```python
from build123d import *

# Parameters (mm, degrees)
SKIZZE1_W                        = 266
SKIZZE1_H                        = 80
AUFSATZ_LINEAR_AUSTRAGEN1_DEPTH  = 20
SKIZZE4_R                        = 6.5
SCHNITT_LINEAR_AUSTRAGEN1_DEPTH  = 20
SKIZZE9_R                        = 15
SCHNITT_LINEAR_AUSTRAGEN5_DEPTH  = 16.8
SKIZZE10_W                       = 20
SKIZZE10_H                       = 15
SCHNITT_LINEAR_AUSTRAGEN6_DEPTH  = 24.3
SKIZZE11_W                       = 91.383535354
SKIZZE11_H                       = 106.650454953
SKIZZE11_W_2                     = 30.220228655
SKIZZE11_H_2                     = 75
SCHNITT_LINEAR_AUSTRAGEN7_DEPTH  = 304.3
SKIZZE12_R                       = 24.75
SCHNITT_LINEAR_AUSTRAGEN8_DEPTH  = 3
SKIZZE13_W                       = 20
SKIZZE13_H                       = 20
SCHNITT_LINEAR_AUSTRAGEN10_DEPTH = 20
VERRUNDUNG1_R                    = 3
SKIZZE14_W                       = 20
SKIZZE14_H                       = 20
SCHNITT_LINEAR_AUSTRAGEN11_DEPTH = 20
VERRUNDUNG2_R                    = 3
SKIZZE15_R                       = 2
SCHNITT_LINEAR_AUSTRAGEN12_DEPTH = 20
M5_GEWINDEBOHRUNG1_D             = 4.2
M5_GEWINDEBOHRUNG1_CSINK_D       = 5.05
M5_GEWINDEBOHRUNG1_CSINK_ANGLE   = 90
SCHNITT_LINEAR_AUSTRAGEN13_DEPTH = 30
SCHNITT_LINEAR_AUSTRAGEN14_DEPTH = 6
SKIZZE19_R                       = 3
SCHNITT_LINEAR_AUSTRAGEN15_DEPTH = 20


with BuildPart() as part:
    # Skizze1 → Aufsatz-Linear austragen1 (new body)
    with BuildSketch(Plane.XY):
        with Locations((43.523698588, -6.755674232)):
            Rectangle(SKIZZE1_W, SKIZZE1_H)
    extrude(amount=AUFSATZ_LINEAR_AUSTRAGEN1_DEPTH)

    # Skizze4 → Schnitt-Linear austragen1 (cut)
    with BuildSketch(Plane(origin=(0, 0, 0), x_dir=(-1, 0, 0), z_dir=(0, 0, -1))):
        with Locations((-43.523698588, -6.755674232)):
            Circle(SKIZZE4_R)
    extrude(amount=-SCHNITT_LINEAR_AUSTRAGEN1_DEPTH, mode=Mode.SUBTRACT)

    # Skizze9 → Schnitt-Linear austragen5 (cut)
    with BuildSketch(Plane(origin=(0, 0, 0), x_dir=(-1, 0, 0), z_dir=(0, 0, -1))):
        with Locations((-43.523698588, -6.755674232)):
            Circle(SKIZZE9_R)
    extrude(amount=-SCHNITT_LINEAR_AUSTRAGEN5_DEPTH, mode=Mode.SUBTRACT)

    # Skizze10 → Schnitt-Linear austragen6 (cut)
    with BuildSketch(Plane.XY.offset(20)):
        with Locations((-79.476301412, 25.744325768)):
            Rectangle(SKIZZE10_W, SKIZZE10_H)
        with Locations((-79.476301412, -39.255674232)):
            Rectangle(SKIZZE10_W, SKIZZE10_H)
        with Locations((166.523698588, -39.255674232)):
            Rectangle(SKIZZE10_W, SKIZZE10_H)
        with Locations((166.523698588, 25.744325768)):
            Rectangle(SKIZZE10_W, SKIZZE10_H)
    extrude(amount=-SCHNITT_LINEAR_AUSTRAGEN6_DEPTH, mode=Mode.SUBTRACT)

    # Skizze11 → Schnitt-Linear austragen7 (cut)
    with BuildSketch(Plane.ZY.offset(89.476301412)):
        with Locations((10.152146704, -6.755674232)):
            Rectangle(SKIZZE11_W, SKIZZE11_H)
        with Locations((10.152146705, -6.755674232)):
            Rectangle(SKIZZE11_W_2, SKIZZE11_H_2, mode=Mode.SUBTRACT)
    extrude(amount=-SCHNITT_LINEAR_AUSTRAGEN7_DEPTH, mode=Mode.SUBTRACT)

    # Skizze12 → Schnitt-Linear austragen8 (cut)
    with BuildSketch(Plane(origin=(0, 0, 0), x_dir=(-1, 0, 0), z_dir=(0, 0, -1))):
        with Locations((-43.523698588, -6.755674232)):
            Circle(SKIZZE12_R)
    extrude(amount=-SCHNITT_LINEAR_AUSTRAGEN8_DEPTH, mode=Mode.SUBTRACT)

    # Skizze13 → Schnitt-Linear austragen10 (cut)
    with BuildSketch(Plane.ZY.offset(89.476301412)):
        with Locations((10, -6.755674232)):
            Rectangle(SKIZZE13_W, SKIZZE13_H)
    extrude(amount=-SCHNITT_LINEAR_AUSTRAGEN10_DEPTH, mode=Mode.SUBTRACT)

    # Verrundung1
    verrundung1_edges = [part.edges().sort_by_distance(p)[0] for p in [
        (-69.476301412, 3.244325768, 10),
        (-69.476301412, -16.755674232, 10),
        (-69.476301412, -31.755674232, 10),
        (-69.476301412, 18.244325768, 10),
    ]]
    fillet(verrundung1_edges, radius=VERRUNDUNG1_R)

    # Skizze14 → Schnitt-Linear austragen11 (cut)
    with BuildSketch(Plane(origin=(176.523698588, 0, 0), x_dir=(0, 0, -1), z_dir=(1, 0, 0))):
        with Locations((-10, -6.755674232)):
            Rectangle(SKIZZE14_W, SKIZZE14_H)
    extrude(amount=-SCHNITT_LINEAR_AUSTRAGEN11_DEPTH, mode=Mode.SUBTRACT)

    # Verrundung2
    verrundung2_edges = [part.edges().sort_by_distance(p)[0] for p in [
        (156.523698588, 3.244325768, 10),
        (156.523698588, -16.755674232, 10),
        (156.523698588, 18.244325768, 10),
        (156.523698588, -31.755674232, 10),
    ]]
    fillet(verrundung2_edges, radius=VERRUNDUNG2_R)

    # Skizze15 → Schnitt-Linear austragen12 (cut)
    with BuildSketch(Plane(origin=(0, 0, 0), x_dir=(-1, 0, 0), z_dir=(0, 0, -1))):
        with Locations((79.476301412, 10.744325768)):
            Circle(SKIZZE15_R)
        with Locations((79.476301412, -24.255674232)):
            Circle(SKIZZE15_R)
        with Locations((-166.523698588, 10.744325768)):
            Circle(SKIZZE15_R)
        with Locations((-166.523698588, -24.255674232)):
            Circle(SKIZZE15_R)
    extrude(amount=-SCHNITT_LINEAR_AUSTRAGEN12_DEPTH, mode=Mode.SUBTRACT)

    # M5 Gewindebohrung1 (through all)
    with Locations(Plane(origin=(166.523698588, 10.744325768, 0), x_dir=(-1, 0, 0), z_dir=(0, 0, -1))):
        with Locations((0, 0), (0, -35), (246, 0), (246, -35)):
            CounterSinkHole(M5_GEWINDEBOHRUNG1_D / 2, M5_GEWINDEBOHRUNG1_CSINK_D / 2, counter_sink_angle=M5_GEWINDEBOHRUNG1_CSINK_ANGLE)

    # Skizze17 → Schnitt-Linear austragen13 (cut)
    with BuildSketch(Plane(origin=(0, 0, 0), x_dir=(-1, 0, 0), z_dir=(0, 0, -1))):
        with BuildLine():
            Line((-149.773698588, -12.255674232), (-149.773698588, -15.255674232))
            ThreePointArc((-149.773698588, -15.255674232), (-151.523698588, -17.005674232), (-153.273698588, -15.255674232))
            Line((-153.273698588, -15.255674232), (-153.273698588, -12.255674232))
            ThreePointArc((-153.273698588, -12.255674232), (-151.523698588, -10.505674232), (-149.773698588, -12.255674232))
        make_face()
        with BuildLine():
            Line((-74.773698588, -12.255674232), (-74.773698588, -15.255674232))
            ThreePointArc((-74.773698588, -15.255674232), (-76.523698588, -17.005674232), (-78.273698588, -15.255674232))
            Line((-78.273698588, -15.255674232), (-78.273698588, -12.255674232))
            ThreePointArc((-78.273698588, -12.255674232), (-76.523698588, -10.505674232), (-74.773698588, -12.255674232))
        make_face()
        with BuildLine():
            Line((-74.773698588, -32.255674232), (-74.773698588, -35.255674232))
            ThreePointArc((-74.773698588, -35.255674232), (-76.523698588, -37.005674232), (-78.273698588, -35.255674232))
            Line((-78.273698588, -35.255674232), (-78.273698588, -32.255674232))
            ThreePointArc((-78.273698588, -32.255674232), (-76.523698588, -30.505674232), (-74.773698588, -32.255674232))
        make_face()
        with BuildLine():
            Line((-149.773698588, -32.255674232), (-149.773698588, -35.255674232))
            ThreePointArc((-149.773698588, -35.255674232), (-151.523698588, -37.005674232), (-153.273698588, -35.255674232))
            Line((-153.273698588, -35.255674232), (-153.273698588, -32.255674232))
            ThreePointArc((-153.273698588, -32.255674232), (-151.523698588, -30.505674232), (-149.773698588, -32.255674232))
        make_face()
    extrude(amount=-SCHNITT_LINEAR_AUSTRAGEN13_DEPTH, mode=Mode.SUBTRACT)

    # Skizze18 → Schnitt-Linear austragen14 (cut)
    with BuildSketch(Plane(origin=(0, 0, 0), x_dir=(-1, 0, 0), z_dir=(0, 0, -1))):
        with BuildLine():
            Line((-148.523698588, -9.718914621), (-148.523698588, -18.718914621))
            ThreePointArc((-148.523698588, -18.718914621), (-151.523698588, -21.718914621), (-154.523698588, -18.718914621))
            Line((-154.523698588, -18.718914621), (-154.523698588, -9.718914621))
            ThreePointArc((-154.523698588, -9.718914621), (-151.523698588, -6.718914621), (-148.523698588, -9.718914621))
        make_face()
        with BuildLine():
            Line((-148.523698588, -29.255674232), (-148.523698588, -38.255674232))
            ThreePointArc((-148.523698588, -38.255674232), (-151.523698588, -41.255674232), (-154.523698588, -38.255674232))
            Line((-154.523698588, -38.255674232), (-154.523698588, -29.255674232))
            ThreePointArc((-154.523698588, -29.255674232), (-151.523698588, -26.255674232), (-148.523698588, -29.255674232))
        make_face()
        with BuildLine():
            Line((-73.523698588, -9.255674232), (-73.523698588, -18.255674232))
            ThreePointArc((-73.523698588, -18.255674232), (-76.523698588, -21.255674232), (-79.523698588, -18.255674232))
            Line((-79.523698588, -18.255674232), (-79.523698588, -9.255674232))
            ThreePointArc((-79.523698588, -9.255674232), (-76.523698588, -6.255674232), (-73.523698588, -9.255674232))
        make_face()
        with BuildLine():
            Line((-73.523698588, -29.255674232), (-73.523698588, -38.255674232))
            ThreePointArc((-73.523698588, -38.255674232), (-76.523698588, -41.255674232), (-79.523698588, -38.255674232))
            Line((-79.523698588, -38.255674232), (-79.523698588, -29.255674232))
            ThreePointArc((-79.523698588, -29.255674232), (-76.523698588, -26.255674232), (-73.523698588, -29.255674232))
        make_face()
    extrude(amount=-SCHNITT_LINEAR_AUSTRAGEN14_DEPTH, mode=Mode.SUBTRACT)

    # Skizze19 → Schnitt-Linear austragen15 (cut)
    with BuildSketch(Plane(origin=(0, 0, 0), x_dir=(-1, 0, 0), z_dir=(0, 0, -1))):
        with Locations((16.476301412, -6.755674232)):
            Circle(SKIZZE19_R)
        with Locations((-103.523698588, -6.755674232)):
            Circle(SKIZZE19_R)
    extrude(amount=-SCHNITT_LINEAR_AUSTRAGEN15_DEPTH, mode=Mode.SUBTRACT)


solid = part.part
```
Design review of the part built by this model. Coordinates are the model's own, in mm. A direction names the side the tool comes from. Coordinates: 2 decimals unless noted, no trailing zeros. Order: outer loops, then holes, each group sorted by start corner. A loop starts at its lowest first (then second) coordinate and runs counter-clockwise, first axis right, second up.
1) Clearance check with flat-ended pins moving along their axes: pin 1 (1.8 mm diameter, centred on y = -13.5, z = 2.5, fed in from +X); pin 2 (3 mm diameter, centred on x = 150.5, y = -30, fed in from -Z); pin 3 (2.5 mm diameter, centred on y = -14, z = 12, fed in from +X). State where each tip first meets the part, or that it passes through.
2) For faces 5 (the flat face through (-69.476, 26, 10)), 6 (the flat face through (156.524, 26, 10)), 7 (the flat face through (168, -31.756, 10)), 8 (the flat face through (79.524, -34, 3)), list the 3-axis set-ups (+Z, -Z, +X, -X, +Y, -Y) from which the entire face can be reached by the end or side of a thin tool; tool diameter is ignored.
3) Take a section at A-A, the plane x = 41. Give the boundary of the cut face in (y, z).
4) Wall thickness on line 1 along X through (y, z) = (-35, 1); line 2 along X through (y, z) = (-8, 14.75); line 3 along X through (y, z) = (-8.5, 4.5): over which ranges is each line inside the solid? List them lowest first.
5) Mouldability with a two-part tool opening along X and no side actions: class faces 1 (the flat face through (-69.476, -7, 10)), 2 (the flat face through (42, 19, 0)), 3 (the cylindrical face through (-81.574, 10.837, 10.35)), 4 (the flat face through (176.524, 11, 10)) as +X half, -X half, draft (parallel to the pull), parting line (faces both ways), or undercut.
Returned:
1. pin 1: stops at x = 156.59
1. pin 2: stops at z = 6
1. pin 3: stops at x = 156.92
2. face 5: +Z, -Z, -X, +Y
2. face 6: +Z, -Z, +X, +Y
2. face 7: +Z, -Z, +X, -Y
2. face 8: -Z
3. outline: (-44.26, 0) - (-31.38, 0) - (-31.38, 3) - (-21.54, 3) - (-21.54, 16.8) - (-12.75, 16.8) - (-12.75, 20) - (-44.26, 20) - close; (-0.77, 16.8) - (8.03, 16.8) - (8.03, 3) - (17.87, 3) - (17.87, 0) - (30.74, 0) - (30.74, 20) - (-0.77, 20) - close
4. line 1: x = -69.48 to 73.52, 79.52 to 148.52, 154.52 to 156.52
4. line 2: x = -69.48 to -19.21, -13.75 to 28.58, 58.47 to 100.79, 106.25 to 156.52
4. line 3: x = -69.48 to -18.92, -14.04 to 28.63, 58.42 to 73.62, 79.43 to 101.08, 105.96 to 148.78, 154.26 to 156.52
5. face 1: -X half
5. face 2: draft
5. face 3: undercut
5. face 4: +X half
